Could you check a few things on this model? Use its own coordinates, in mm. Give positions to 0.01 mm unless a question says otherwise; leave off trailing zeros. Order: outer loops, then holes, each group sorted by start corner. A loop starts at its lowest first (then second) coordinate and runs counter-clockwise, first axis right, second up.
(1) If I drill on probe 1 along X at (y, z) = (0, -1.25); probe 2 along Y at (x, z) = (23, 1.5); probe 3 along Y at (x, z) = (27.25, 0), over which ranges is the centre line in solid material (lowest first)?
(2) Imagine slicing it at C-C, the plane x = 12.5. Write out the boundary of the cut face in (y, z).
(3) Imagine slicing it at B-B, the plane y = -2.25. Write out the boundary of the cut face in (x, z), then the cut area to 3 significant figures.
(4) Will this pin go through, and if not, where does the flat tip stop? pin 1 (3 mm diameter, centred on x = 23, y = 0, fed in from +Z).
(5) Imagine slicing it at A-A, the plane x = 23. Write out the boundary of the cut face in (y, z), then the cut area to 3 significant figures.
Autodesk Inventor part; units mm, degrees
ref_plane "YZ Plane" through (0, 0, 0) normal (1, 0, 0) x (0, 1, 0)
ref_plane "XZ Plane" through (0, 0, 0) normal (0, 1, 0) x (-1, 0, 0)
ref_plane "XY Plane" through (0, 0, 0) normal (0, 0, 1) x (1, 0, 0)
sketch "Sketch1" plane through (0, 0, 0) normal (0, 1, 0) x (-1, 0, 0)
  line L0 (-30, -7.5) -> (30, -7.5)
  line L1 (30, -7.5) -> (30, 7.5)
  line L2 (30, 7.5) -> (-30, 7.5)
  line L3 (-30, 7.5) -> (-30, -7.5)
  line L4 (-30, -7.5) -> (30, 7.5) construction
  line L5 (30, -7.5) -> (-30, 7.5) construction
  point P0 (0, 0)
  dimension "d0" = 15
  dimension "d1" = 60
extrude "Extrusion1" add sketch "Sketch1" along normal mid plane 8
sketch "Sketch2" plane through (0, 4, 0) normal (0, 1, 0) x (1, 0, 0)
  line L0 (30, 7.5) -> (-30, 7.5)
  line L1 (-30, 7.5) -> (-30, -7.5)
  line L2 (-30, -7.5) -> (30, -7.5)
  line L3 (30, -7.5) -> (30, 7.5)
  line L4 (-30, -7.5) -> (30, -7.5)
  line L5 (10, -7.5) -> (30, -5.5)
  line L6 (30, -7.5) -> (30, 7.5)
  point P0 (0, 0)
  dimension "d4" = 20
  dimension "d5" = 2
extrude "Extrusion2" cut sketch "Sketch2" against normal through all contours L3 L2 L5
mirror "Mirror1" about plane through (0, 0, 0) normal (0, 0, 1) of "Extrusion2"
fillet "Fillet1" radius 2 6 edges at (-30, 0, 7.5) (-30, 0, -7.5) (10, 0, -7.5) (10, 0, 7.5) (30, 0, 5.5) (30, 0, -5.5)
sketch "Sketch3" plane through (30, -4, 3.69) normal (1, 0, 0) x (0, 0, -1)
  line L0 (7.38, 8) -> (7.38, 0)
  line L1 (0, 8) -> (7.38, 8)
  line L2 (0, 0) -> (0, 8)
  line L3 (7.38, 0) -> (0, 0)
  line L4 (7.38, 8) -> (0, 8)
  line L5 (0, 8) -> (0, 0)
  line L6 (0, 0) -> (7.38, 0)
  line L7 (7.38, 0) -> (7.38, 8)
  line L8 (7.38, 8) -> (0, 0) construction
  line L9 (0, 8) -> (7.38, 0) construction
  point P0 (3.69, 4)
  point P1 (3.69, 4)
hole "Hole1" at (30, 0, 0) direction (-1, 0, 0) diameter 2 depth 8 tip angle 118
sketch "Sketch4" plane through (-28, -4, 7.5) normal (0, 0, 1) x (1, 0, 0)
  line L0 (58, 0) -> (58, 8)
  point P0 (28, 4)
  point P1 (51, 4)
  point P2 (58, 4)
  dimension "d16" = 7
hole "Hole2" at (23, 0, 7.5) direction (0, 0, -1) diameter 2.459 end through all
properties part number "Switch_Extend"
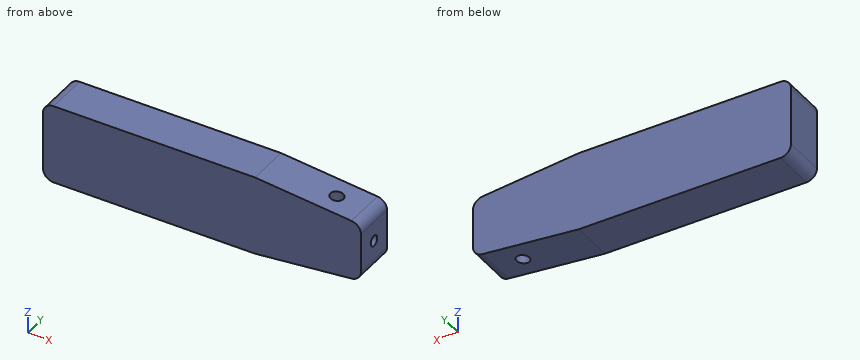
Answer block:
1. probe 1: x = -30 to 21.77, 24.23 to 30
1. probe 2: y = -4 to -1.23, 1.23 to 4
1. probe 3: y = -4 to -1, 1 to 4
2. outline: (-4, -7.25) - (4, -7.25) - (4, 7.25) - (-4, 7.25) - close
3. outline: (-30, -5.5) arc R2 ccw to (-28, -7.5) - (10, -7.5) - (28.2, -5.68) arc R2 ccw to (30, -3.69) - (30, 3.69) arc R2 ccw to (28.2, 5.68) - (10, 7.5) - (-28, 7.5) arc R2 ccw to (-30, 5.5) - close
3. area: 857 mm2
4. pin 1: stops at z = 6.35
5. outline: (-4, -6.2) - (-1.23, -6.2) - (-1.23, 6.2) - (-4, 6.2) - close; (1.23, -6.2) - (4, -6.2) - (4, 6.2) - (1.23, 6.2) - close
5. area: 68.7 mm2
